Could you check a few things on this model? Use its own coordinates, in mm. Face numbers are marked on the shaded views. A direction names the side the tool comes from. Round coordinates to 2 decimals unless told otherwise and drop trailing zeros. Write each loop counter-clockwise with the first axis right and the second up, starting at its lowest first coordinate (ties: lowest second). Pieces come first, ordered by that corner, then holes. Notation, with made-up numbers: M -5.5,19 L 14.5,19 A22 cw 14.5,37 Z; hole C -32,-7.5 d8. An arc over 180 degrees is marked long. One line per item, written item: value. Start each with the question number.
(1) I'm going to push flat-ended pins straight in: pin 1 Ø1.5 at (y, z) = (-3.5, 2) entering from -X; pin 2 Ø0.9 at (y, z) = (-1, 1) entering from -X; pin 3 Ø1.5 at (x, z) = (25.5, 1.5) entering from -Y. Where does each tip first touch, or does it pass through?
(2) I want a section at B-B on y = 14.5. Please give me the cut outline in (x, z).
(3) Which directions (+Z, -Z, +X, -X, +Y, -Y) give clear straight access to the entire face, cutting with the end or side of a thin tool? Please do the marked faces 1, 2 and 3.
(4) I want a section at C-C on x = 10. Please give me the cut outline in (y, z).
(5) If I drill on L1, parallel to Y at x = -7.5, z = 1; L2, parallel to Y at x = 8, z = 1.2; L3, parallel to X at y = 16, z = 0.5, over which ranges is the centre line in solid material (lowest first)?
(6) I want a section at A-A on z = 1.2. Please give me the cut outline in (x, y).
Autodesk Inventor part; units mm, degrees
ref_plane "YZ Plane" through (0, 0, 0) normal (1, 0, 0) x (0, 1, 0)
ref_plane "XZ Plane" through (0, 0, 0) normal (0, 1, 0) x (-1, 0, 0)
ref_plane "XY Plane" through (0, 0, 0) normal (0, 0, 1) x (1, 0, 0)
sketch "Sketch1" plane through (0, 0, 0) normal (0, 0, 1) x (1, 0, 0)
  line L0 (-7.2302, -2.2309) -> (-2.2302, -2.2309)
  line L1 (-2.2302, -2.2309) -> (-2.2302, -5.2309)
  line L2 (-2.2302, -5.2309) -> (7.7698, -5.2309)
  line L3 (7.7698, -5.2309) -> (7.7698, -2.2309)
  line L4 (7.7698, -2.2309) -> (12.7698, -2.2309)
  line L5 (-7.2302, -2.2309) -> (-7.2302, 2.7691)
  line L6 (-7.2302, 2.7691) -> (-10.2302, 2.7691)
  line L7 (-10.2302, 2.7691) -> (-10.2302, 12.7691)
  line L8 (-10.2302, 12.7691) -> (-7.2302, 12.7691)
  line L9 (-7.2302, 12.7691) -> (-7.2302, 17.7691)
  line L10 (-7.2302, 17.7691) -> (12.7698, -2.2309)
  point P0 (0, 0)
  dimension "d2" = 5
  dimension "d3" = 5
  dimension "d4" = 10
  dimension "d5" = 5
  dimension "d6" = 10
  dimension "d7" = 5
extrude "Extrusion1" add sketch "Sketch1" along normal blind 3
sketch "Sketch2" plane through (0, 0, 3) normal (0, 0, 1) x (1, 0, 0)
  line L0 (-7.2302, 17.7691) -> (-7.2302, 12.7691)
  line L1 (-7.2302, 17.7691) -> (-7.2302, 32.7691)
  line L2 (12.7698, -2.2309) -> (-7.2302, 17.7691)
  line L3 (12.7698, -2.2309) -> (27.7698, -2.2309)
  line L4 (-7.2302, 32.7691) -> (27.7698, -2.2309)
  line L5 (-7.2302, 17.7691) -> (12.7698, -2.2309)
  point P0 (0, 0)
  dimension "d14" = 15
  dimension "d15" = 15
extrude "Extrusion2" add sketch "Sketch2" against normal blind 3
sketch "Sketch3" plane through (-10.2302, 12.7691, 0) normal (0, 1, 0) x (1, 0, 0)
  line L0 (0, 0) -> (0, -3)
  line L1 (3, 0) -> (3, -3)
  line L2 (0, 0) -> (3, 0)
  line L3 (3, 0) -> (3, -3)
  line L4 (3, -3) -> (0, -3)
  line L5 (0, -3) -> (0, 0)
  point P0 (10.2302, 0)
extrude "Extrusion3" add sketch "Sketch3" along normal blind 15
sketch "Sketch4" plane through (7.7698, -5.2309, 0) normal (1, 0, 0) x (0, 0, -1)
  line L0 (-3, 3) -> (-3, 0)
  line L1 (-3, 3) -> (0, 3)
  line L2 (0, 3) -> (0, 0)
  line L3 (0, 0) -> (-3, 0)
  line L4 (-3, 0) -> (-3, 3)
  point P0 (0, 5.2309)
extrude "Extrusion4" add sketch "Sketch4" along normal blind 15
properties part number "Support Piece"
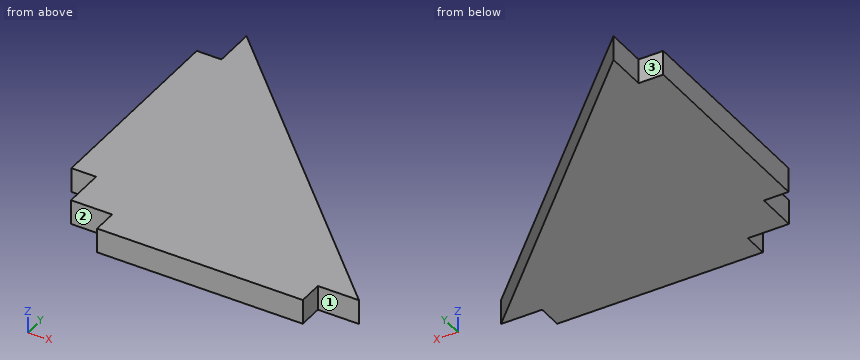
Found:
1. pin 1: stops at x = -2.23
1. pin 2: stops at x = -7.23
1. pin 3: stops at y = -2.23
2. outline: M -10.23,0 L 11.04,0 L 11.04,3 L -10.23,3 Z
3. face 1: +Z, -Z, +X, -Y
3. face 2: +Z, -Z, -X, -Y
3. face 3: +Z, -Z, -X, +Y
4. outline: M -5.23,0 L 15.54,0 L 15.54,3 L -5.23,3 Z
5. L1: y = 2.77 to 27.77
5. L2: y = -5.23 to 17.54
5. L3: x = -10.23 to 9.54
6. outline: M -10.23,2.77 L -7.23,2.77 L -7.23,-2.23 L -2.23,-2.23 L -2.23,-5.23 L 22.77,-5.23 L 22.77,-2.23 L 27.77,-2.23 L -7.23,32.77 L -7.23,27.77 L -10.23,27.77 Z
